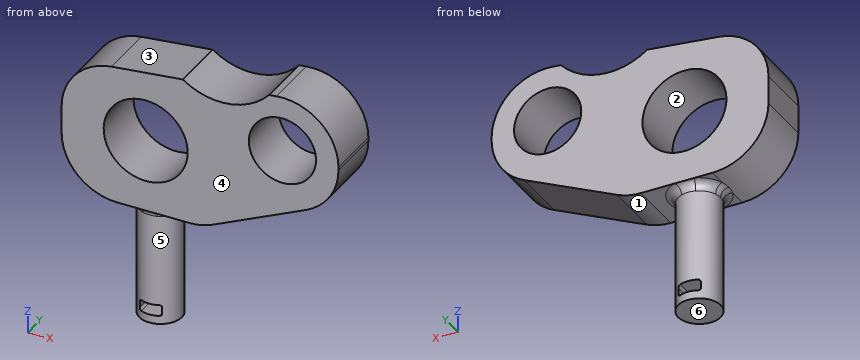
from build123d import *

# Parameters (mm, degrees)
SKETCH1_R           = 5
BOSS_EXTRUDE1_DEPTH = 20
SKETCH2_R           = 5
SKETCH2_R_2         = 3.98
CUT_EXTRUDE2_DEPTH  = 8
SKETCH8_R           = 5
BOSS_EXTRUDE2_DEPTH = 20
BOSS_EXTRUDE3_START = -31.5
BOSS_EXTRUDE3_DEPTH = 31.5
BOSS_EXTRUDE4_START = -31.5
BOSS_EXTRUDE4_DEPTH = 31.5
SKETCH12_R          = 7.5
SKETCH12_R_2        = 6
CUT_EXTRUDE3_DEPTH  = 31.5
CUT_EXTRUDE4_DEPTH  = 55.083269132
FILLET1_R           = 10
BOSS_EXTRUDE5_START = 13
SKETCH17_R          = 3.98
BOSS_EXTRUDE5_DEPTH = 13
CUT_EXTRUDE5_DEPTH  = 52.315568407
SKETCH19_R          = 5
SKETCH19_R_2        = 3.98
CUT_EXTRUDE6_DEPTH  = 0.5
SKETCH20_R          = 3.98
SKETCH20_R_2        = 3.8
CUT_EXTRUDE7_DEPTH  = 21.5
FILLET2_R           = 1.5
CUT_EXTRUDE9_DEPTH  = 10


with BuildPart() as part:
    # Sketch1 → Boss-Extrude1 (new body)
    with BuildSketch(Plane.XY):
        Circle(SKETCH1_R)
    extrude(amount=BOSS_EXTRUDE1_DEPTH)

    # Sketch2 → Cut-Extrude2 (cut)
    with BuildSketch(Plane(origin=(0, 0, 0), x_dir=(-1, 0, 0), z_dir=(0, 0, -1))):
        Circle(SKETCH2_R)
        Circle(SKETCH2_R_2, mode=Mode.SUBTRACT)
    extrude(amount=-CUT_EXTRUDE2_DEPTH, mode=Mode.SUBTRACT)

    # Sketch8 → Boss-Extrude2 (add)
    with BuildSketch(Plane.XY.offset(20)):
        with Locations(Location((0, 0, 0), (0, 0, 180))):
            Circle(SKETCH8_R)
    extrude(amount=BOSS_EXTRUDE2_DEPTH)

    # Sketch9 → Boss-Extrude3 (add)
    with BuildSketch(Plane.XY.offset(40).offset(BOSS_EXTRUDE3_START)):
        with BuildLine():
            Line((0, 5), (35, 5))
            Line((35, 5), (35, -5))
            Line((35, -5), (0, -5))
            ThreePointArc((0, -5), (5, 0), (0, 5))
        make_face()
    extrude(amount=BOSS_EXTRUDE3_DEPTH)

    # Sketch10 → Boss-Extrude4 (add)
    with BuildSketch(Plane.XY.offset(40).offset(BOSS_EXTRUDE4_START)):
        with BuildLine():
            ThreePointArc((0, -5), (-5, 0), (0, 5))
            Line((0, 5), (-15, 5))
            Line((-15, 5), (-15, -5))
            Line((-15, -5), (0, -5))
        make_face()
    extrude(amount=BOSS_EXTRUDE4_DEPTH)

    # Sketch12 → Cut-Extrude3 (cut)
    with BuildSketch(Plane(origin=(0, 5, 0), x_dir=(1, 0, 0), z_dir=(0, 1, 0))):
        with Locations(Location((0, -21.5, 0), (0, 0, 270))):
            Circle(SKETCH12_R)
        with Locations(Location((24.415869627, -26.872644634, 0), (0, 0, 270))):
            Circle(SKETCH12_R_2)
    extrude(amount=-CUT_EXTRUDE3_DEPTH, mode=Mode.SUBTRACT)

    # Sketch14 → Cut-Extrude4 (cut, through all)
    with BuildSketch(Plane(origin=(0, 5, 0), x_dir=(1, 0, 0), z_dir=(0, 1, 0))):
        Polygon((-15, -40), (35, -40), (35, -37.368304137), (35, -8.5), (10, -8.5), (34.415869627, -19.756213623), (34.415869627, -37.872644634), (-15, -32.5), align=None)
    extrude(amount=-CUT_EXTRUDE4_DEPTH, mode=Mode.SUBTRACT)

    # Fillet1
    fillet1_edges = [part.edges().sort_by_distance(p)[0] for p in [
        (-15, 0, 8.5),
        (34.415869627, 0, 19.756213623),
        (10, 0, 8.5),
        (-15, 0, 32.5),
        (34.415869627, 0, 37.872644634),
    ]]
    fillet(fillet1_edges, radius=FILLET1_R - 0.0001)  # a hair under: the kernel refuses the full size

    # Sketch17 → Boss-Extrude5 (add)
    with BuildSketch(Plane(origin=(0, 0, 0), x_dir=(-1, 0, 0), z_dir=(0, 0, -1)).offset(BOSS_EXTRUDE5_START)):
        Circle(SKETCH17_R)
    extrude(amount=-BOSS_EXTRUDE5_DEPTH)

    # Sketch18 → Cut-Extrude5 (cut, through all)
    with BuildSketch(Plane(origin=(0, 5, 0), x_dir=(1, 0, 0), z_dir=(0, 1, 0))):
        with BuildLine():
            Line((-1.6, 11.5), (1.6, 11.5))
            ThreePointArc((1.6, 11.5), (1.882842712, 11.382842712), (2, 11.1))
            Line((2, 11.1), (2, 9.9))
            ThreePointArc((2, 9.9), (1.882842712, 9.617157288), (1.6, 9.5))
            Line((1.6, 9.5), (-1.6, 9.5))
            ThreePointArc((-1.6, 9.5), (-1.882842712, 9.617157288), (-2, 9.9))
            Line((-2, 9.9), (-2, 11.1))
            ThreePointArc((-2, 11.1), (-1.882842712, 11.382842712), (-1.6, 11.5))
        make_face()
    extrude(amount=-CUT_EXTRUDE5_DEPTH, mode=Mode.SUBTRACT)

    # Sketch19 → Cut-Extrude6 (cut)
    with BuildSketch(Plane(origin=(0, 0, 8), x_dir=(-1, 0, 0), z_dir=(0, 0, -1))):
        Circle(SKETCH19_R)
        Circle(SKETCH19_R_2, mode=Mode.SUBTRACT)
    extrude(amount=-CUT_EXTRUDE6_DEPTH, mode=Mode.SUBTRACT)

    # Sketch20 → Cut-Extrude7 (cut)
    with BuildSketch(Plane(origin=(0, 0, -13), x_dir=(-1, 0, 0), z_dir=(0, 0, -1))):
        Circle(SKETCH20_R)
        Circle(SKETCH20_R_2, mode=Mode.SUBTRACT)
    extrude(amount=-CUT_EXTRUDE7_DEPTH, mode=Mode.SUBTRACT)

    # Fillet2
    fillet2_edges = [part.edges().sort_by_distance(p)[0] for p in [
        (3.8, 0, 8.5),
    ]]
    fillet(fillet2_edges, radius=FILLET2_R)

    # Sketch21 → Cut-Extrude9 (cut)
    with BuildSketch(Plane.XZ.offset(5)):
        with BuildLine():
            Line((22.038458054, 36.526934554), (6.637283612, 34.852471718))
            ThreePointArc((6.637283612, 34.852471718), (14.662129167, 32.707278529), (22.038458054, 36.526934554))
        make_face()
    extrude(amount=-CUT_EXTRUDE9_DEPTH, mode=Mode.SUBTRACT)


solid = part.part
Work out the finished part from the listing and answer in its coordinate system (mm). Face numbers are marked on the shaded views. A direction names the side the tool comes from. Coordinates: 2 decimals unless noted, no trailing zeros. Loops run counter-clockwise (first coordinate to the right, second up) from the corner with the lowest first, then second, coordinate; pieces in that order, holes last. Notation, with made-up numbers: (-6.75, 48) -> (44.25, 48) arc R29 ccw to (44.25, 86) -> close; hole circle Ø11 at (23, 67.25). An arc over 180 degrees is marked (long way). Answer as CSV lines item,"result".
1) For the marked faces 5 and 6, determine the directions among +Z, -Z, +X, -X, +Y, -Y from which every point of the face is accessible in a straight line to the end or side of a thin tool.
A:
face 5,"-Z"
face 6,"-Z, +X, -X, +Y, -Y"
2) For a pull along Z with two mould halves and no side action, classify the marked faces 1, 2, 3 and 4 as released by +Z, released by -Z, zero draft, split by the parting line, or undercut.
A:
face 1,"released by -Z"
face 2,"undercut"
face 3,"released by +Z"
face 4,"zero draft"
3) Straight lines are drawn through the part: probe 1 along X at (y, z) = (3.5, 27); probe 2 along X at (y, z) = (-1.5, 23); probe 3 along X at (y, z) = (-1, 32). For each, find the intervals that lie inside material, in ascending order.
A:
probe 1,"x = -14.38 to -5.1, 5.1 to 18.42, 30.41 to 34.41"
probe 2,"x = -15 to -7.35, 7.35 to 19.83, 29 to 33.9"
probe 3,"x = -10.31 to 21.3, 27.53 to 32.91"
4) The part is cut by section D-D (z = -1). Give the vertices of the cut face in (x, y).
A:
outline,"circle Ø7.6 at (0, 0)"
5) Flat-ended cylindrical pins translate along their axes: pin 1 (5 mm diameter, centred on x = 2.5, z = 25, fed in from -Y); pin 2 (0.6 mm diameter, centred on y = 0.5, z = -10.5, fed in from +X); pin 3 (5 mm diameter, centred on y = 1, z = 19, fed in from +X) (3 decimals); pin 4 (1 mm diameter, centred on x = 7, y = 2, fed in from -Z). Find the tip coordinate at first contact, or state that the pin passes through.
A:
pin 1,"passes through"
pin 2,"stops at x = 3.79"
pin 3,"stops at x = 33.265"
pin 4,"stops at z = 8.5"
6) The part is cut by section A-A (z = 21.5). Give the vertices of the cut face in (x, y).
A:
outline,"(-15, -5) -> (-7.5, -5) -> (-7.5, 5) -> (-15, 5) -> close; (7.5, -5) -> (21.74, -5) -> (21.74, 5) -> (7.5, 5) -> close; (27.09, -5) -> (33.27, -5) -> (33.27, 5) -> (27.09, 5) -> close"
7) The part is cut by section B-B (x = 29.5). Give the vertices of the cut face in (y, z).
A:
outline,"(-5, 17.55) -> (5, 17.55) -> (5, 23.69) -> (-5, 23.69) -> close; (-5, 30.06) -> (5, 30.06) -> (5, 35.34) -> (-5, 35.34) -> close"
8) The part is cut by section C-C (z = 16). Give the vertices of the cut face in (x, y).
A:
outline,"(-14.68, -5) -> (-5.1, -5) -> (-5.1, 5) -> (-14.68, 5) -> close; (5.1, -5) -> (26.27, -5) -> (26.27, 5) -> (5.1, 5) -> close"
